Autodesk Inventor part; units mm, degrees
ref_plane "YZ Plane" through (0, 0, 0) normal (1, 0, 0) x (0, 1, 0)
ref_plane "XZ Plane" through (0, 0, 0) normal (0, 1, 0) x (-1, 0, 0)
ref_plane "XY Plane" through (0, 0, 0) normal (0, 0, 1) x (1, 0, 0)
sketch "Sketch1" plane through (0, 0, 0) normal (0, 0, 1) x (1, 0, 0)
  line L0 (0, 0) -> (35, 0)
  line L1 (35, 0) -> (35, 45)
  line L2 (0, 45) -> (35, 45) construction
  circle A0 centre (4.5, 40.5) radius 1.25
  line L3 (17.5, 50) -> (17.5, 0) construction
  circle A1 centre (30.5, 40.5) radius 1.25
  line L4 (0, 45) -> (0, 0)
  line L5 (0, 22.5) -> (35, 22.5) construction
  circle A2 centre (4.5, 4.5) radius 1.25
  circle A3 centre (30.5, 4.5) radius 1.25
  line L6 (8.5, 3.5) -> (26.5, 3.5)
  line L7 (26.5, 3.5) -> (26.5, 43.5)
  line L8 (26.5, 43.5) -> (8.5, 43.5)
  line L9 (8.5, 43.5) -> (8.5, 3.5)
  line L10 (8.5, 3.5) -> (10, 3.5)
  line L11 (8.5, 4.5) -> (8.5, 3.5)
  line L12 (9.5, 4.5) -> (9.5, 43.5)
  line L13 (8.5, 4.5) -> (11, 4.5)
  line L14 (11, 4.5) -> (11, 3.5)
  line L15 (25.5, 4.5) -> (25.5, 43.5)
  line L16 (26.5, 4.5) -> (24, 4.5)
  line L17 (24, 4.5) -> (24, 3.5)
  line L18 (0, 45) -> (35, 45)
  line L19 (0, 45) -> (0, 0)
  point P0 (11, 4)
  point P1 (24, 4)
  point P2 (9.5, 4.5)
  point P3 (25.5, 4.5)
  point P4 (24, 3.5)
  dimension "d5" = 2.5
  dimension "d6" = 4.5
  dimension "d8" = 2.5
  dimension "d9" = 18
  dimension "d10" = 40
  dimension "d11" = 3.5
  dimension "d19" = 1
  dimension "d26" = 8
  dimension "d27" = 2.5
  dimension "d28" = 35
  dimension "d29" = 1.5
  dimension "d30" = 26
  dimension "d31" = 9
  dimension "d54" = 45
extrude "Extrusion1" add sketch "Sketch1" along normal blind 2 contours L4 L18 L1 L0 | L9 L13 L14 L6 | L9 L8 L12 L13 | L14 L13 L12 L8 L15 L16 L17 L6 | L17 L16 L7 L6 | L8 L7 L16 L15
extrude "Extrusion2" add sketch "Sketch1" against normal blind 8 contours L9 L13 L14 L6 | L9 L8 L12 L13 | L17 L16 L7 L6 | L8 L7 L16 L15
fillet "Fillet1" radius 2 2 edges at (26.5, 3.5, -4) (8.5, 3.5, -4)
fillet "Fillet2" radius 2 2 edges at (25.5, 43.5, -4) (9.5, 43.5, -4)
fillet "Fillet3" radius 2 4 edges at (35, 45, 1) (0, 45, 1) (0, 0, 1) (35, 0, 1)
thicken "Thicken1" operation add thickness 8 both sides no extend neighbours no toward (0, 0, -1) faces at (19.6667, 29.3453, 0)
sketch "Sketch3" plane through (33, 0, -8) normal (0, 0, -1) x (-1, 0, 0)
  line L0 (15, 49) -> (15, -1) construction
  line L1 (-2.5, 20) -> (32.5, 20) construction
  line L2 (6, 2.5) -> (24, 2.5)
  line L3 (24, 2.5) -> (24, 42.5)
  line L4 (24, 42.5) -> (6, 42.5)
  line L5 (6, 42.5) -> (6, 2.5)
  line L6 (6, 2.5) -> (7.5, 2.5)
  line L7 (6, 3.5) -> (6, 2.5)
  line L8 (7, 3.5) -> (7, 42.5)
  line L9 (6, 3.5) -> (8.5, 3.5)
  line L10 (8.5, 3.5) -> (8.5, 2.5)
  line L11 (23, 3.5) -> (23, 42.5)
  line L12 (24, 3.5) -> (21.5, 3.5)
  line L13 (21.5, 3.5) -> (21.5, 2.5)
  line L14 (31, 0) -> (0, 0)
  point P0 (33, 0)
  point P1 (8.5, 3)
  point P2 (21.5, 3)
  point P3 (7, 3.5)
  dimension "d36" = 18
  dimension "d37" = 40
  dimension "d38" = 1
  dimension "d39" = 8
  dimension "d40" = 2.5
  dimension "d41" = 9
  dimension "d42" = 2.5
  dimension "d43" = 7
  dimension "d44" = 8.5
extrude "Extrusion3" cut sketch "Sketch3" against normal blind 8 contours L10 L9 L8 L4 L11 L12 L13 L2
sketch "Sketch4" plane through (0, 0, 2) normal (0, 0, 1) x (1, 0, 0)
  line L0 (10, 42.5) -> (10, 3.5)
  line L1 (5, 45) -> (10, 45)
  line L2 (10, 45) -> (10, 38)
  line L3 (10, 38) -> (3, 38)
  line L4 (3, 38) -> (3, 43)
  line L5 (33, 45) -> (28, 45)
  line L6 (28, 45) -> (28, 38)
  line L7 (28, 38) -> (35, 38)
  line L8 (35, 38) -> (35, 43)
  arc A0 (5, 45) -> (3, 43) centre (5, 43) ccw
  arc A1 (35, 43) -> (33, 45) centre (33, 43) ccw
  line L9 (0, 0) -> (0, 45)
  line L10 (35, 2) -> (35, 43)
  line L11 (35, 22.5) -> (39, 22.5)
  line L12 (10, 2.5) -> (10, 41.5)
  line L13 (5, 0) -> (10, 0)
  line L14 (10, 0) -> (10, 7)
  line L15 (10, 7) -> (3, 7)
  line L16 (3, 7) -> (3, 2)
  line L17 (33, 0) -> (28, 0)
  line L18 (28, 0) -> (28, 7)
  line L19 (28, 7) -> (35, 7)
  line L20 (35, 7) -> (35, 2)
  arc A2 (3, 2) -> (5, 0) centre (5, 2) ccw
  arc A3 (33, 0) -> (35, 2) centre (33, 2) ccw
  line L21 (0, 45) -> (0, 0)
  line L22 (35, 43) -> (35, 2)
  point P0 (35, 45)
  point P1 (35, 0)
  point P2 (35, 7)
  point P3 (0, 10)
  point P4 (0, 2)
  dimension "d47" = 7
  dimension "d48" = 2
  dimension "d49" = 2
extrude "Extrusion4" cut sketch "Sketch4" against normal blind 8
sketch "Sketch6" plane through (11.5, 2.5, -8) normal (0, 1, 0) x (1, 0, 0)
  line L0 (23.5, -10) -> (16.5, -10)
  line L1 (14.5, 0) -> (-1.5, 0)
  line L2 (16.5, -10) -> (-1.5, -10)
  line L3 (-1.5, -10) -> (-1.5, 0)
  line L4 (-1.5, 0) -> (16.5, 0)
  line L5 (16.5, 0) -> (16.5, -10)
  point P0 (-11.5, -8)
  point P1 (13.5, 0)
extrude "Extrusion5" [suppressed]
properties part number "Sensor Housing"
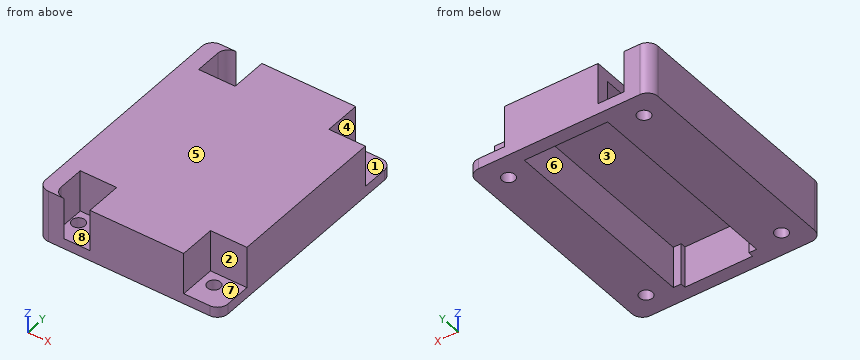
Design review of the part built by this model. Coordinates are the model's own, in mm. Face numbers are marked on the shaded views. A direction names the side the tool comes from. Coordinates: 2 decimals unless noted, no trailing zeros. Write each loop counter-clockwise with the first axis right and the second up, starting at its lowest first coordinate (ties: lowest second). Pieces come first, ordered by that corner, then holes. Notation, with made-up numbers: M -32.75,-16.75 L -8.75,-16.75 A14 ccw -8.75,-9.75 Z; hole C 59.25,58 d3. An arc over 180 degrees is marked long. Answer as a JSON object with one key per item and string values.
Item 1: Add section D-D, the plane y = 40.5. Give the boundary of the cut face in (x, z), and give its area (3 significant figures).
Outcome:
{"outline": "M 0,-8 L 3.25,-8 L 3.25,-6 L 3,-6 L 3,2 L 0,2 Z; M 5.75,-8 L 10,-8 L 10,-6 L 5.75,-6 Z; M 10,0 L 26,0 L 26,-8 L 29.25,-8 L 29.25,-6 L 28,-6 L 28,2 L 10,2 Z; M 31.75,-8 L 35,-8 L 35,-6 L 31.75,-6 Z", "area": "100 mm²"}
Item 2: Add section B-B, the plane y = 6.5. Give the boundary of the cut face in (x, z), and give its area (3 significant figures).
Outcome:
{"outline": "M 0,-8 L 10,-8 L 10,-6 L 3,-6 L 3,2 L 0,2 Z; M 10,0 L 26,0 L 26,-8 L 35,-8 L 35,-6 L 28,-6 L 28,2 L 10,2 Z", "area": "110 mm²"}
Item 3: Insertion check: pin 1 Ø2 at (x, z) = (5.5, -3.5) entering from +Y; pin 2 Ø2 at (x, z) = (31.5, 0) entering from -Y; pin 3 Ø3.5 at (x, y) = (31, 2.5) entering from +Z; pin 4 Ø2 at (x, y) = (30.5, 4.5) entering from +Z. Each pin has a flat end and moves straight along its axis. Give the tip position at first contact, or say it passes through.
Outcome:
{"pin 1": "y = 45", "pin 2": "y = 7", "pin 3": "z = -6", "pin 4": "through"}
Item 4: Add section C-C, the plane z = -7. Give the boundary of the cut face in (x, y).
Outcome:
{"outline": "M 0,2 A2 ccw 2,0 L 33,0 A2 ccw 35,2 L 35,43 A2 ccw 33,45 L 2,45 A2 ccw 0,43 Z; hole C 4.5,4.5 d2.5; hole C 4.5,40.5 d2.5; hole M 10,3.5 L 11.5,3.5 L 11.5,2.5 L 24.5,2.5 L 24.5,3.5 L 26,3.5 L 26,42.5 L 10,42.5 Z; hole C 30.5,4.5 d2.5; hole C 30.5,40.5 d2.5"}
Item 5: Draft analysis for pull direction Y (two halves, no side actions). For the marked faces 1, 2 and 3, state which applies: pulls with the +Y half, pulls with the -Y half, needs draft (parallel to the pull), parting line crosses it, or undercut.
Outcome:
{"face 1": "needs draft", "face 2": "pulls with the -Y half", "face 3": "undercut"}
Item 6: Add section A-A, the plane z = -1.5. Give the boundary of the cut face in (x, y), and give its area (3 significant figures).
Outcome:
{"outline": "M 0,2 A2 ccw 2,0 L 5,0 A2 cw 3,2 L 3,7 L 10,7 L 10,38 L 3,38 L 3,43 A2 cw 5,45 L 2,45 A2 ccw 0,43 Z; M 10,0 L 28,0 L 28,7 L 35,7 L 35,38 L 28,38 L 28,45 L 10,45 L 10,42.5 L 26,42.5 L 26,3.5 L 24.5,3.5 L 24.5,2.5 L 11.5,2.5 L 11.5,3.5 L 10,3.5 Z", "area": "742 mm²"}
Item 7: Wall thickness on probe 1 along Y at (x, z) = (4.5, -7); probe 2 along X at (y, z) = (4, -4.5); probe 3 along Y at (x, z) = (19, -2): over which ranges is each line inside the solid? List them lowest first.
Outcome:
{"probe 1": "0 to 3.25, 5.75 to 39.25, 41.75 to 45", "probe 2": "0 to 3, 26 to 28", "probe 3": "0 to 2.5, 42.5 to 45"}
Item 8: Machinability: for the marked faces 4, 5, 6, 7 and 8, which of the approach directions +Z, -Z, +X, -X, +Y, -Y give a long, thin tool a straight path to every point of the face, cutting with its end or side? Answer none if there is none.
Outcome:
{"face 4": "+Z, +X, +Y", "face 5": "+Z, +X, -X, +Y, -Y", "face 6": "-Z", "face 7": "+Z, +X, -Y", "face 8": "+Z"}
